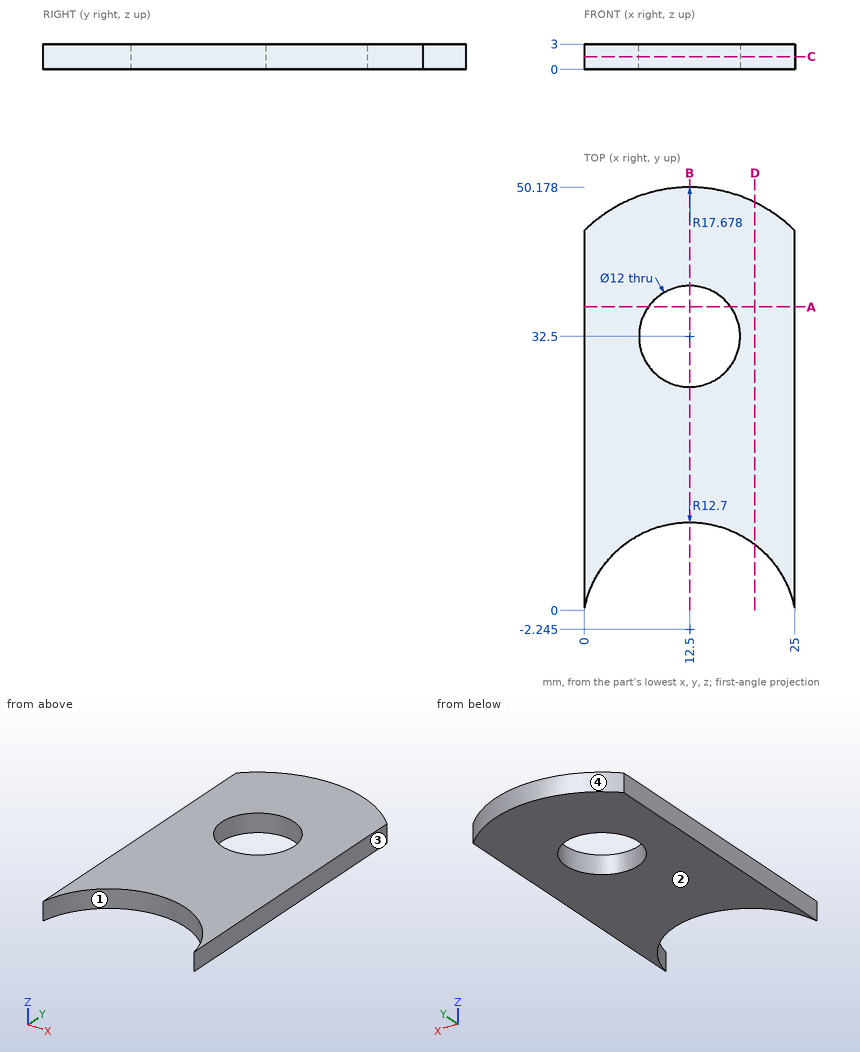
Study the drawing (mm; zero at the part's minimum x, y, z) and answer. Coordinates: 2 decimals unless noted, no trailing zeros. Order: outer loops, then holes, each group sorted by start corner. A loop starts at its lowest first (then second) coordinate and runs counter-clockwise, first axis right, second up. Notation, with made-up numbers: (-37.5, -23.5) -> (-2.5, -23.5) arc R17 ccw to (-2.5, 0.5) -> close; hole circle Ø2 at (-8, 41). An arc over 180 degrees is marked (long way). Answer in a Markdown table with one row per item. Add a question column.
Item 1: Find section C-C (z = 1.5). Write down the section's boundary in (x, y) (1 decimal).
Item 2: Find section D-D (x = 20.25). Write down the section's boundary in (y, z), then the cut area to 3 significant figures.
Item 3: Find the intervals of material crossed by L1, parallel to Y at x = 12.5, z = 2.3 (1 decimal); L2, parallel to X at y = 34, z = 1.45; L3, parallel to X at y = 33.5, z = 0.85, in increasing order. Write a range as from..to.
Item 4: Find section B-B (x = 12.5). Write down the section's boundary in (y, z) (1 decimal).
Item 5: Determine the mould class of the marked faces 1, 2, 3 and 4 for opening direction X: +X half, -X half, draft (parallel to the pull), parting line (faces both ways), or undercut.
Item 6: Find section A-A (y = 36). Write down the section's boundary in (x, z).
Result set:
| question | item | result |
|---|---|---|
| 1 | outline | (0, 0) arc R12.7 cw to (25, 0) -> (25, 45) arc R17.7 ccw to (0, 45) -> close; hole circle Ø12 at (12.5, 32.5) |
| 2 | outline | (7.82, 0) -> (48.39, 0) -> (48.39, 3) -> (7.82, 3) -> close |
| 2 | area | 122 mm² |
| 3 | L1 | y = 10.5..26.5, 38.5..50.2 |
| 3 | L2 | x = 0..6.69, 18.31..25 |
| 3 | L3 | x = 0..6.58, 18.42..25 |
| 4 | outline | (10.5, 0) -> (26.5, 0) -> (26.5, 3) -> (10.5, 3) -> close; (38.5, 0) -> (50.2, 0) -> (50.2, 3) -> (38.5, 3) -> close |
| 5 | face 1 | undercut |
| 5 | face 2 | draft |
| 5 | face 3 | +X half |
| 5 | face 4 | parting line |
| 6 | outline | (0, 0) -> (7.63, 0) -> (7.63, 3) -> (0, 3) -> close; (17.37, 0) -> (25, 0) -> (25, 3) -> (17.37, 3) -> close |
